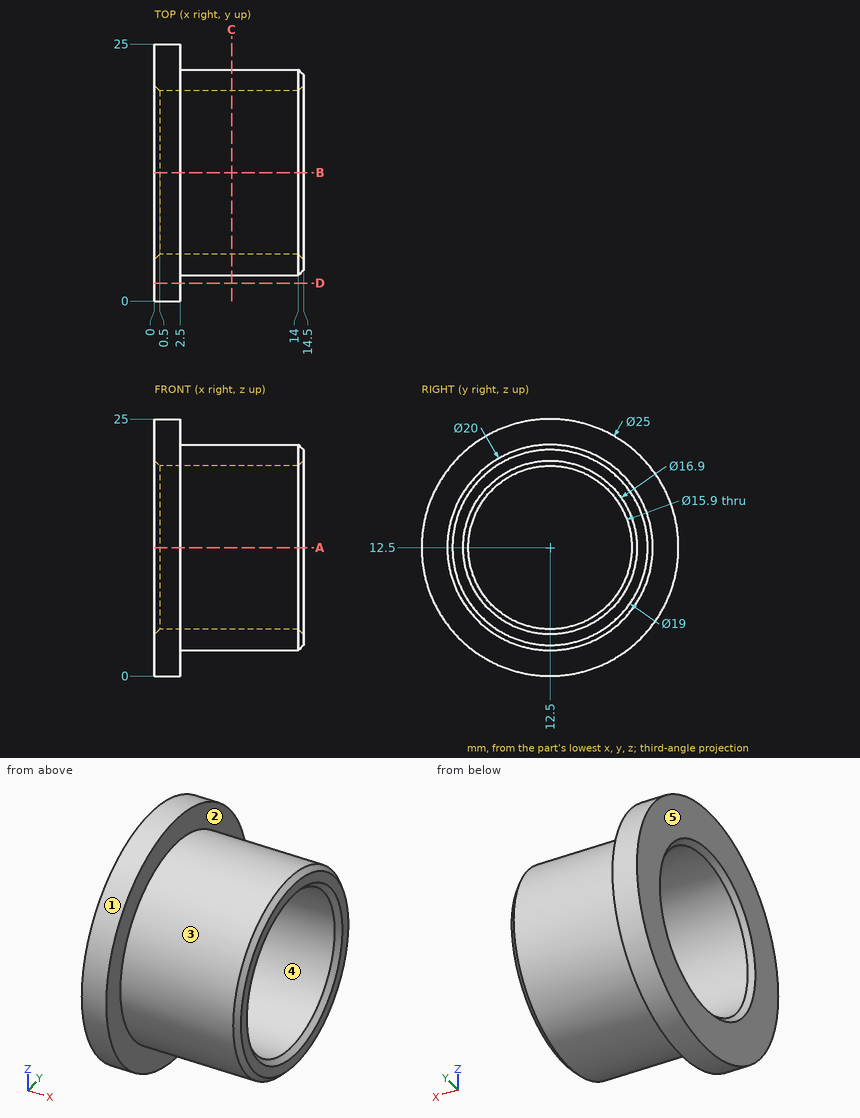
Job drawing, mm, ordinate dimensions from the low corner. One solid piece. A direction names the side the tool comes from. Coordinates: 2 decimals unless noted, no trailing zeros. Order: outer loops, then holes, each group sorted by start corner. A loop starts at its lowest first (then second) coordinate and runs counter-clockwise, first axis right, second up. Notation, with made-up numbers: (57.5, 10) -> (99.5, 10) arc R15 cw to (99.5, 20) -> close; hole circle Ø11 at (10, 36). An arc over 180 degrees is marked (long way). Answer in a Markdown table with one row per item. Add a question column.
Q1. Band-saw the part on D-D, the plane y = 1.75. List the corners of the cut face in (x, z), then the cut area to 3 significant figures.
Q2. Mould opens along Y. For the marked faces 3, 4 and 5 say: +Y half, -Y half, draft (parallel to the pull), parting line (faces both ways), or undercut.
Q3. Band-saw the part on A-A, the plane z = 12.5. List the corners of the cut face in (x, y).
Q4. Wall check: line 1 along Y through (x, z) = (3.75, 12.75); line 2 along X through (y, z) = (17.25, 21.75); line 3 along Z through (x, y) = (3.25, 8.25). Give the ranges that are in metal, low to high. Write a range as [from, to].
Q5. Which spindle directions (+Z, -Z, +X, -X, +Y, -Y) get a long thin tool onto all of the face, cutting with end or side? Do the marked faces 1 and 2. Say none if no direction does.
Q6. Band-saw the part on C-C, the plane x = 7.5. List the corners of the cut face in (y, z), then the cut area to 3 significant figures.
Q7. Drop flat-ended pins along their axis: pin 1 (6 mm diameter, centred on x = 13, y = 10.5, fed in from -Z); pin 2 (5 mm diameter, centred on x = 9.5, z = 14, fed in from +Y); pin 3 (8 mm diameter, centred on x = 8, z = 20, fed in from +Y). Give the stop position or say it passes through.
Answers follow:
| question | item | result |
|---|---|---|
| 1 | outline | (0, 6.12) -> (2.5, 6.12) -> (2.5, 18.88) -> (0, 18.88) -> close |
| 1 | area | 31.9 mm^2 |
| 2 | face 3 | parting line |
| 2 | face 4 | undercut |
| 2 | face 5 | draft |
| 3 | outline | (0, 0) -> (2.5, 0) -> (2.5, 2.5) -> (14, 2.5) -> (14.5, 3) -> (14.5, 4.05) -> (14, 4.55) -> (0.5, 4.55) -> (0, 4.05) -> close; (0, 20.95) -> (0.5, 20.45) -> (14, 20.45) -> (14.5, 20.95) -> (14.5, 22) -> (14, 22.5) -> (2.5, 22.5) -> (2.5, 25) -> (0, 25) -> close |
| 4 | line 1 | [2.5, 4.55], [20.45, 22.5] |
| 4 | line 2 | [0, 2.5] |
| 4 | line 3 | [3.45, 5.78], [19.22, 21.55] |
| 5 | face 1 | +X, -X |
| 5 | face 2 | +X |
| 6 | outline | circle Ø20 at (12.5, 12.5); hole circle Ø15.9 at (12.5, 12.5) |
| 6 | area | 116 mm^2 |
| 7 | pin 1 | z = 2.5 |
| 7 | pin 2 | y = 22.5 |
| 7 | pin 3 | y = 21.87 |
